The listing builds one solid part. Answer for the finished solid, in the listing's coordinates (mm). Face numbers are marked on the shaded views. A direction names the side the tool comes from. Give positions to 0.01 mm unless a question says otherwise; leave off trailing zeros. Order: outer loops, then holes, each group sorted by start corner. A loop starts at its lowest first (then second) coordinate and runs counter-clockwise, first axis right, second up. Notation, with made-up numbers: M 70,80 L 123,80 A25 ccw 123,93 Z; hole C -32,-37 d6. An arc over 180 degrees is marked long. Answer as a JSON object with one key per item and string values. Group by question number.
```python
from build123d import *

# Parameters (mm, degrees)
ESQUISSE1_R                  = 1.75
BOSS_EXTRU_1_DEPTH           = 2
ESQUISSE2_R                  = 1.3
ESQUISSE2_R_2                = 2.4
ENL_V_MAT_EXTRU_1_DEPTH      = 1
ENL_V_MAT_EXTRU_1_DEPTH_BACK = 5


with BuildPart() as part:
    # Esquisse1 → Boss.-Extru.1 (new body, symmetric)
    with BuildSketch(Plane.XY):
        with BuildLine():
            ThreePointArc((30.75, -4), (34.75, 0), (30.75, 4))
            Line((30.75, 4), (11.409123542, 4))
            ThreePointArc((11.409123542, 4), (11.194344337, 4.566700654), (10.951436862, 5.12192646))
            ThreePointArc((10.951436862, 5.12192646), (12.008090957, 5.965388247), (12.82210701, 7.044889767))
            ThreePointArc((12.82210701, 7.044889767), (12.669951657, 7.315), (12.51210701, 7.581825517))
            ThreePointArc((12.51210701, 7.581825517), (11.170223244, 7.416617696), (9.911436862, 6.9232593))
            ThreePointArc((9.911436862, 6.9232593), (9.591641884, 7.359925677), (9.252623584, 7.781841479))
            ThreePointArc((9.252623584, 7.781841479), (10.05496909, 8.870045207), (10.561852666, 10.123446462))
            ThreePointArc((10.561852666, 10.123446462), (10.344972209, 10.344972209), (10.123446462, 10.561852666))
            ThreePointArc((10.123446462, 10.561852666), (8.870045207, 10.05496909), (7.781841479, 9.252623584))
            ThreePointArc((7.781841479, 9.252623584), (7.359925677, 9.591641884), (6.9232593, 9.911436862))
            ThreePointArc((6.9232593, 9.911436862), (7.416617696, 11.170223244), (7.581825517, 12.51210701))
            ThreePointArc((7.581825517, 12.51210701), (7.315, 12.669951657), (7.044889767, 12.82210701))
            ThreePointArc((7.044889767, 12.82210701), (5.965388247, 12.008090957), (5.12192646, 10.951436862))
            ThreePointArc((5.12192646, 10.951436862), (4.626642697, 11.169703548), (4.122086336, 11.365584201))
            ThreePointArc((4.122086336, 11.365584201), (4.272836063, 12.709169027), (4.085109489, 14.048088143))
            ThreePointArc((4.085109489, 14.048088143), (3.78652263, 14.131494839), (3.486235477, 14.208555951))
            ThreePointArc((3.486235477, 14.208555951), (2.654199937, 13.14288127), (2.112960617, 11.903927815))
            ThreePointArc((2.112960617, 11.903927815), (1.578061664, 11.986568374), (1.04, 12.04518576))
            ThreePointArc((1.04, 12.04518576), (0.837867713, 13.382005944), (0.31, 14.626715284))
            ThreePointArc((0.31, 14.626715284), (0, 14.63), (-0.31, 14.626715284))
            ThreePointArc((-0.31, 14.626715284), (-0.837867713, 13.382005944), (-1.04, 12.04518576))
            ThreePointArc((-1.04, 12.04518576), (-1.578061664, 11.986568374), (-2.112960617, 11.903927815))
            ThreePointArc((-2.112960617, 11.903927815), (-2.654199937, 13.14288127), (-3.486235477, 14.208555951))
            ThreePointArc((-3.486235477, 14.208555951), (-3.78652263, 14.131494839), (-4.085109489, 14.048088143))
            ThreePointArc((-4.085109489, 14.048088143), (-4.272836063, 12.709169027), (-4.122086336, 11.365584201))
            ThreePointArc((-4.122086336, 11.365584201), (-4.626642697, 11.169703548), (-5.12192646, 10.951436862))
            ThreePointArc((-5.12192646, 10.951436862), (-5.965388247, 12.008090957), (-7.044889767, 12.82210701))
            ThreePointArc((-7.044889767, 12.82210701), (-7.315, 12.669951657), (-7.581825517, 12.51210701))
            ThreePointArc((-7.581825517, 12.51210701), (-7.416617696, 11.170223244), (-6.9232593, 9.911436862))
            ThreePointArc((-6.9232593, 9.911436862), (-7.359925677, 9.591641884), (-7.781841479, 9.252623584))
            ThreePointArc((-7.781841479, 9.252623584), (-8.870045207, 10.05496909), (-10.123446462, 10.561852666))
            ThreePointArc((-10.123446462, 10.561852666), (-10.344972209, 10.344972209), (-10.561852666, 10.123446462))
            ThreePointArc((-10.561852666, 10.123446462), (-10.05496909, 8.870045207), (-9.252623584, 7.781841479))
            ThreePointArc((-9.252623584, 7.781841479), (-9.591641884, 7.359925677), (-9.911436862, 6.9232593))
            ThreePointArc((-9.911436862, 6.9232593), (-11.170223244, 7.416617696), (-12.51210701, 7.581825517))
            ThreePointArc((-12.51210701, 7.581825517), (-12.669951657, 7.315), (-12.82210701, 7.044889767))
            ThreePointArc((-12.82210701, 7.044889767), (-12.008090957, 5.965388247), (-10.951436862, 5.12192646))
            ThreePointArc((-10.951436862, 5.12192646), (-11.169703548, 4.626642697), (-11.365584201, 4.122086336))
            ThreePointArc((-11.365584201, 4.122086336), (-12.709169027, 4.272836063), (-14.048088143, 4.085109489))
            ThreePointArc((-14.048088143, 4.085109489), (-14.131494839, 3.78652263), (-14.208555951, 3.486235477))
            ThreePointArc((-14.208555951, 3.486235477), (-13.14288127, 2.654199937), (-11.903927815, 2.112960617))
            ThreePointArc((-11.903927815, 2.112960617), (-11.986568374, 1.578061664), (-12.04518576, 1.04))
            ThreePointArc((-12.04518576, 1.04), (-13.382005944, 0.837867713), (-14.626715284, 0.31))
            ThreePointArc((-14.626715284, 0.31), (-14.63, 0), (-14.626715284, -0.31))
            ThreePointArc((-14.626715284, -0.31), (-13.382005944, -0.837867713), (-12.04518576, -1.04))
            ThreePointArc((-12.04518576, -1.04), (-11.986568374, -1.578061664), (-11.903927815, -2.112960617))
            ThreePointArc((-11.903927815, -2.112960617), (-13.14288127, -2.654199937), (-14.208555951, -3.486235477))
            ThreePointArc((-14.208555951, -3.486235477), (-14.131494839, -3.78652263), (-14.048088143, -4.085109489))
            ThreePointArc((-14.048088143, -4.085109489), (-12.709169027, -4.272836063), (-11.365584201, -4.122086336))
            ThreePointArc((-11.365584201, -4.122086336), (0.064808849, -12.089826294), (11.409123542, -4))
            Line((11.409123542, -4), (30.75, -4))
        make_face()
        with Locations((30.75, 0)):
            Circle(ESQUISSE1_R, mode=Mode.SUBTRACT)
        Circle(ESQUISSE1_R, mode=Mode.SUBTRACT)
    extrude(amount=BOSS_EXTRU_1_DEPTH, both=True)

    # Esquisse2 → Enlèv. mat.-Extru.1 (cut, two sides)
    with BuildSketch(Plane.XY.offset(2)) as enl_v_mat_extru_1_sk:
        with Locations((4.5, 0)):
            Circle(ESQUISSE2_R)
        with Locations((-4.5, 0)):
            Circle(ESQUISSE2_R)
        Circle(ESQUISSE2_R_2)
    extrude(amount=ENL_V_MAT_EXTRU_1_DEPTH, mode=Mode.SUBTRACT)
    extrude(enl_v_mat_extru_1_sk.sketch, amount=-ENL_V_MAT_EXTRU_1_DEPTH_BACK, mode=Mode.SUBTRACT)


solid = part.part
```
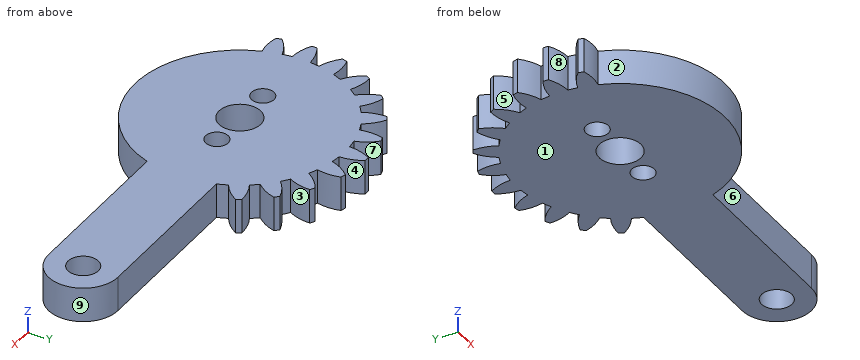
Item 1: Section A-A (z = 0.9) is taken. Count the separate pieces of the cut face and the enclosed holes in it, and give its area (3 significant figures).
Item 2: Consider probe 1 along X at (y, z) = (10, 0.4); probe 2 along Y at (x, z) = (0, -0.8); probe 3 along Y at (x, z) = (30.75, 1.2). Determine where each line is inside the solid, lowest interval first. Write a range as from..to.
Item 3: Determine the mould class of the marked faces 6, 7, 8 and 9 for opening direction X: released by +X, released by -X, zero draft, split by the parting line, or undercut.
Item 4: A tool of negligible diameter and unlimited length cuts with its end or side. For the marked faces 1, 2, 3, 4 and 5, from which of +Z, -Z, +X, -X, +Y, -Y can it reach the whole face along a straight path? Write none if from no direction.
Item 5: Section B-B (x = 20) is taken. Determine the outline of the cut face in (y, z).
Item 6: Flat-ended cylindrical pins translate along their axes: P1, Ø3, axis at x = 30.75, y = 0, coming from the -Z side; P2, Ø2, axis at x = 23.5, z = 1, coming from the +Y side; P3, Ø1.5, axis at y = 6, z = -1, coming from the +X side; P4, Ø1.5, axis at x = 10.5, z = -1, coming from the +Y side. Find the tip coordinate at first contact, or state that the pin passes through.
Values found:
{
 "1": {"separate pieces": "1", "enclosed holes": "4", "area": "645 mm^2"},
 "2": {"probe 1": "x = -10.53..-8.77, -6.97..6.97, 8.77..10.53", "probe 2": "y = -12.09..-2.4, 2.4..14.63", "probe 3": "y = -4..-1.75, 1.75..4"},
 "3": {"face 6": "zero draft", "face 7": "undercut", "face 8": "released by -X", "face 9": "released by +X"},
 "4": {"face 1": "-Z, +X, -X, +Y, -Y", "face 2": "+Z, -Z, -Y", "face 3": "+Z, -Z", "face 4": "+Z, -Z, +Y", "face 5": "+Z, -Z, -X"},
 "5": {"outline": "M -4,-2 L 4,-2 L 4,2 L -4,2 Z"},
 "6": {"P1": "passes through", "P2": "stops at y = 4", "P3": "stops at x = 12.64", "P4": "stops at y = 10.56"}
}
